Input: part model. Units: mm. Frame: model coordinates. Round coordinates to 2 decimals unless told otherwise and drop trailing zeros. Loops run counter-clockwise (first coordinate to the right, second up) from the corner with the lowest first, then second, coordinate; pieces in that order, holes last. Notation, with made-up numbers: M -12.75,9 L 31.25,9 A14 cw 31.25,26 Z; hole C 79,52 d3. An arc over 180 degrees is marked long. Put each result on its own line as item: value. Start each with the question number.
1) Line query: probe 1 along Z at (x, y) = (4.75, 5.5); probe 2 along X at (y, z) = (0.75, -12); probe 3 along Z at (x, y) = (10.25, 1.25). Output: solid intervals per line, ascending.
2) Draft query along Z for faces 1 (the face through (8, 3, -17.729)), 2 (the face through (11.087, 3.194, -13.286)), 3 (the face through (8, 3, 0)), 4 (the face through (6.7, 6.299, -6.8)). Return one class per face: +Z half, -Z half, draft (parallel to the pull), parting line (faces both ways), or undercut.
3) Section B-B on x = 6. Output: boundary loops of the cut face in (y, z).
4) Section A-A on z = -16. Output: boundary loops of the cut face in (x, y), plus the area to 3 significant figures.
5) Section C-C on y = 4. Output: boundary loops of the cut face in (x, z), plus the area to 3 significant figures.
6) Section D-D on z = -11.5. Output: boundary loops of the cut face in (x, y), plus the area to 3 significant figures.
from build123d import *

# Parameters (mm, degrees)
SKETCH1_W                          = 15.8496
SKETCH1_H                          = 6.2992
BASE_EXTRUDE_DEPTH                 = 17.7292
F_5_16_18_TAPPED_HOLE1_D           = 6.5278
F_5_16_18_TAPPED_HOLE1_CBORE_D     = 7.9375
F_5_16_18_TAPPED_HOLE1_CBORE_DEPTH = 15.875
CHAMFER1_SIZE                      = 2.54


with BuildPart() as part:
    # Sketch1 → Base-Extrude (new body)
    with BuildSketch(Plane.XY):
        with Locations((7.9248, 3.1496)):
            Rectangle(SKETCH1_W, SKETCH1_H)
    extrude(amount=-BASE_EXTRUDE_DEPTH)

    # 5/16-18 Tapped Hole1 (through all)
    with Locations(Plane(origin=(0, 6.2992, 0), x_dir=(-1, 0, 0), z_dir=(0, 1, 0))):
        with Locations((-7.9375, -10.8712)):
            CounterBoreHole(F_5_16_18_TAPPED_HOLE1_D / 2, F_5_16_18_TAPPED_HOLE1_CBORE_D / 2, F_5_16_18_TAPPED_HOLE1_CBORE_DEPTH)

    # Chamfer1
    chamfer1_edges = [part.edges().sort_by_distance(p)[0] for p in [
        (0, 6.2992, -8.8646),
        (15.8496, 6.2992, -8.8646),
    ]]
    chamfer(chamfer1_edges, length=CHAMFER1_SIZE)


solid = part.part
Geometry results:
1. probe 1: z = -17.73 to -13.24, -8.51 to 0
1. probe 2: x = 0 to 4.13, 11.74 to 15.85
1. probe 3: z = -17.73 to -14.1, -7.65 to 0
2. face 1: -Z half
2. face 2: undercut
2. face 3: +Z half
2. face 4: draft
3. outline: M 0,-17.73 L 6.3,-17.73 L 6.3,-14.33 L 0,-14.33 Z; M 0,-7.41 L 6.3,-7.41 L 6.3,0 L 0,0 Z
4. outline: M 0,0 L 15.85,0 L 15.85,3.76 L 13.31,6.3 L 2.54,6.3 L 0,3.76 Z
4. area: 93.4 mm²
5. outline: M 0.24,-17.73 L 15.61,-17.73 L 15.61,0 L 0.24,0 Z; hole C 7.94,-10.87 d7.94
5. area: 223 mm²
6. outline: M 0,0 L 4.02,0 L 4.02,6.3 L 2.54,6.3 L 0,3.76 Z; M 11.86,0 L 15.85,0 L 15.85,3.76 L 13.31,6.3 L 11.86,6.3 Z
6. area: 44.0 mm²
